Could you check a few things on this model? Use its own coordinates, in mm. Coordinates: 2 decimals unless noted, no trailing zeros. Order: outer loops, then holes, each group sorted by start corner. A loop starts at its lowest first (then second) coordinate and runs counter-clockwise, first axis right, second up. Notation, with made-up numbers: (-14, 52.25) -> (8, 52.25) arc R15 cw to (8, 81.25) -> close; hole circle Ø5 at (-23.5, 28). An arc over 180 degrees is marked (long way). Use a Markdown table: item, result. Add a question column.
1) If we section it at B-B (z = 2.65): Write out the boundary of the cut face in (x, y).
2) If we section it at A-A (x = 0): Write out the boundary of the cut face in (y, z), plus the area to 4 significant figures.
3) If we section it at D-D (z = 4.75): Write out the boundary of the cut face in (x, y), plus the area to 3 significant figures.
4) Will these pins go through, and if not, where does the flat tip stop? pin 1 Ø3 at (y, z) = (-12, 2) entering from -X; pin 2 Ø1 at (x, y) = (7, -14.5) entering from +Z.
5) If we section it at C-C (x = 14.5): Write out the boundary of the cut face in (y, z).
6) If I drill on L1, parallel to Y at x = 0, z = 0.6; L2, parallel to Y at x = -9.5, z = 0.35; L3, parallel to Z at x = -17.5, y = 2, over which ranges is the centre line in solid material (lowest first)? Write a range as [from, to].
```python
from build123d import *

# Parameters (mm, degrees)
CROQUIS2_R              = 20
SALIENTE_EXTRUIR2_DEPTH = 1
CROQUIS2_5_R            = 5
SALIENTE_EXTRUIR3_DEPTH = 5.5
CHAFL_N1_SIZE           = 5
CORTAR_EXTRUIR1_DEPTH   = 29.814059068


with BuildPart() as part:
    # Croquis2 → Saliente-Extruir2 (new body)
    with BuildSketch(Plane.XY):
        Circle(CROQUIS2_R)
        with BuildLine():
            Line((-2.039607805, 0.95), (2.039607805, 0.95))
            ThreePointArc((2.039607805, 0.95), (0, -2.25), (-2.039607805, 0.95))
        make_face(mode=Mode.SUBTRACT)
        with BuildLine():
            Line((-0.854679553, 13.973887178), (-1.098873712, 17.966426372))
            ThreePointArc((-1.098873712, 17.966426372), (0, 18), (1.098873712, 17.966426372))
            Line((1.098873712, 17.966426372), (0.854679553, 13.973887178))
            ThreePointArc((0.854679553, 13.973887178), (0, 14), (-0.854679553, 13.973887178))
        make_face(mode=Mode.SUBTRACT)
        with BuildLine():
            Line((-3.58862282, 17.638644683), (-2.791151082, 13.718945865))
            ThreePointArc((-2.791151082, 13.718945865), (-3.623466631, 13.522961568), (-4.44226519, 13.276531173))
            Line((-4.44226519, 13.276531173), (-5.711483815, 17.069825794))
            ThreePointArc((-5.711483815, 17.069825794), (-4.658742812, 17.386664873), (-3.58862282, 17.638644683))
        make_face(mode=Mode.SUBTRACT)
        with BuildLine():
            Line((-8.031560636, 16.108818509), (-6.246769384, 12.529081062))
            ThreePointArc((-6.246769384, 12.529081062), (-7, 12.124355653), (-7.727117794, 11.674401509))
            Line((-7.727117794, 11.674401509), (-9.934865736, 15.009944797))
            ThreePointArc((-9.934865736, 15.009944797), (-9, 15.588457268), (-8.031560636, 16.108818509))
        make_face(mode=Mode.SUBTRACT)
        with BuildLine():
            Line((-11.927160868, 13.481202974), (-9.276680675, 10.485380091))
            ThreePointArc((-9.276680675, 10.485380091), (-9.899494937, 9.899494937), (-10.485380091, 9.276680675))
            Line((-10.485380091, 9.276680675), (-13.481202974, 11.927160868))
            ThreePointArc((-13.481202974, 11.927160868), (-12.727922061, 12.727922061), (-11.927160868, 13.481202974))
        make_face(mode=Mode.SUBTRACT)
        with BuildLine():
            Line((-15.009944797, 9.934865736), (-11.674401509, 7.727117794))
            ThreePointArc((-11.674401509, 7.727117794), (-12.124355653, 7), (-12.529081062, 6.246769384))
            Line((-12.529081062, 6.246769384), (-16.108818509, 8.031560636))
            ThreePointArc((-16.108818509, 8.031560636), (-15.588457268, 9), (-15.009944797, 9.934865736))
        make_face(mode=Mode.SUBTRACT)
        with BuildLine():
            Line((-17.069825794, 5.711483815), (-13.276531173, 4.44226519))
            ThreePointArc((-13.276531173, 4.44226519), (-13.522961568, 3.623466631), (-13.718945865, 2.791151082))
            Line((-13.718945865, 2.791151082), (-17.638644683, 3.58862282))
            ThreePointArc((-17.638644683, 3.58862282), (-17.386664873, 4.658742812), (-17.069825794, 5.711483815))
        make_face(mode=Mode.SUBTRACT)
        with BuildLine():
            Line((-17.966426372, 1.098873712), (-13.973887178, 0.854679553))
            ThreePointArc((-13.973887178, 0.854679553), (-14, 0), (-13.973887178, -0.854679553))
            Line((-13.973887178, -0.854679553), (-17.966426372, -1.098873712))
            ThreePointArc((-17.966426372, -1.098873712), (-18, 0), (-17.966426372, 1.098873712))
        make_face(mode=Mode.SUBTRACT)
        with BuildLine():
            Line((-17.638644683, -3.58862282), (-13.718945865, -2.791151082))
            ThreePointArc((-13.718945865, -2.791151082), (-13.522961568, -3.623466631), (-13.276531173, -4.44226519))
            Line((-13.276531173, -4.44226519), (-17.069825794, -5.711483815))
            ThreePointArc((-17.069825794, -5.711483815), (-17.386664873, -4.658742812), (-17.638644683, -3.58862282))
        make_face(mode=Mode.SUBTRACT)
        with BuildLine():
            Line((-16.108818509, -8.031560636), (-12.529081062, -6.246769384))
            ThreePointArc((-12.529081062, -6.246769384), (-12.124355653, -7), (-11.674401509, -7.727117794))
            Line((-11.674401509, -7.727117794), (-15.009944797, -9.934865736))
            ThreePointArc((-15.009944797, -9.934865736), (-15.588457268, -9), (-16.108818509, -8.031560636))
        make_face(mode=Mode.SUBTRACT)
        with BuildLine():
            Line((-13.481202974, -11.927160868), (-10.485380091, -9.276680675))
            ThreePointArc((-10.485380091, -9.276680675), (-9.899494937, -9.899494937), (-9.276680675, -10.485380091))
            Line((-9.276680675, -10.485380091), (-11.927160868, -13.481202974))
            ThreePointArc((-11.927160868, -13.481202974), (-12.727922061, -12.727922061), (-13.481202974, -11.927160868))
        make_face(mode=Mode.SUBTRACT)
        with BuildLine():
            Line((-9.934865736, -15.009944797), (-7.727117794, -11.674401509))
            ThreePointArc((-7.727117794, -11.674401509), (-7, -12.124355653), (-6.246769384, -12.529081062))
            Line((-6.246769384, -12.529081062), (-8.031560636, -16.108818509))
            ThreePointArc((-8.031560636, -16.108818509), (-9, -15.588457268), (-9.934865736, -15.009944797))
        make_face(mode=Mode.SUBTRACT)
        with BuildLine():
            Line((-5.711483815, -17.069825794), (-4.44226519, -13.276531173))
            ThreePointArc((-4.44226519, -13.276531173), (-3.623466631, -13.522961568), (-2.791151082, -13.718945865))
            Line((-2.791151082, -13.718945865), (-3.58862282, -17.638644683))
            ThreePointArc((-3.58862282, -17.638644683), (-4.658742812, -17.386664873), (-5.711483815, -17.069825794))
        make_face(mode=Mode.SUBTRACT)
        with BuildLine():
            Line((-1.098873712, -17.966426372), (-0.854679553, -13.973887178))
            ThreePointArc((-0.854679553, -13.973887178), (0, -14), (0.854679553, -13.973887178))
            Line((0.854679553, -13.973887178), (1.098873712, -17.966426372))
            ThreePointArc((1.098873712, -17.966426372), (0, -18), (-1.098873712, -17.966426372))
        make_face(mode=Mode.SUBTRACT)
        with BuildLine():
            Line((3.58862282, -17.638644683), (2.791151082, -13.718945865))
            ThreePointArc((2.791151082, -13.718945865), (3.623466631, -13.522961568), (4.44226519, -13.276531173))
            Line((4.44226519, -13.276531173), (5.711483815, -17.069825794))
            ThreePointArc((5.711483815, -17.069825794), (4.658742812, -17.386664873), (3.58862282, -17.638644683))
        make_face(mode=Mode.SUBTRACT)
        with BuildLine():
            Line((8.031560636, -16.108818509), (6.246769384, -12.529081062))
            ThreePointArc((6.246769384, -12.529081062), (7, -12.124355653), (7.727117794, -11.674401509))
            Line((7.727117794, -11.674401509), (9.934865736, -15.009944797))
            ThreePointArc((9.934865736, -15.009944797), (9, -15.588457268), (8.031560636, -16.108818509))
        make_face(mode=Mode.SUBTRACT)
        with BuildLine():
            Line((11.927160868, -13.481202974), (9.276680675, -10.485380091))
            ThreePointArc((9.276680675, -10.485380091), (9.899494937, -9.899494937), (10.485380091, -9.276680675))
            Line((10.485380091, -9.276680675), (13.481202974, -11.927160868))
            ThreePointArc((13.481202974, -11.927160868), (12.727922061, -12.727922061), (11.927160868, -13.481202974))
        make_face(mode=Mode.SUBTRACT)
        with BuildLine():
            Line((15.009944797, -9.934865736), (11.674401509, -7.727117794))
            ThreePointArc((11.674401509, -7.727117794), (12.124355653, -7), (12.529081062, -6.246769384))
            Line((12.529081062, -6.246769384), (16.108818509, -8.031560636))
            ThreePointArc((16.108818509, -8.031560636), (15.588457268, -9), (15.009944797, -9.934865736))
        make_face(mode=Mode.SUBTRACT)
        with BuildLine():
            Line((17.069825794, -5.711483815), (13.276531173, -4.44226519))
            ThreePointArc((13.276531173, -4.44226519), (13.522961568, -3.623466631), (13.718945865, -2.791151082))
            Line((13.718945865, -2.791151082), (17.638644683, -3.58862282))
            ThreePointArc((17.638644683, -3.58862282), (17.386664873, -4.658742812), (17.069825794, -5.711483815))
        make_face(mode=Mode.SUBTRACT)
        with BuildLine():
            Line((17.966426372, -1.098873712), (13.973887178, -0.854679553))
            ThreePointArc((13.973887178, -0.854679553), (14, 0), (13.973887178, 0.854679553))
            Line((13.973887178, 0.854679553), (17.966426372, 1.098873712))
            ThreePointArc((17.966426372, 1.098873712), (18, 0), (17.966426372, -1.098873712))
        make_face(mode=Mode.SUBTRACT)
        with BuildLine():
            Line((17.638644683, 3.58862282), (13.718945865, 2.791151082))
            ThreePointArc((13.718945865, 2.791151082), (13.522961568, 3.623466631), (13.276531173, 4.44226519))
            Line((13.276531173, 4.44226519), (17.069825794, 5.711483815))
            ThreePointArc((17.069825794, 5.711483815), (17.386664873, 4.658742812), (17.638644683, 3.58862282))
        make_face(mode=Mode.SUBTRACT)
        with BuildLine():
            Line((16.108818509, 8.031560636), (12.529081062, 6.246769384))
            ThreePointArc((12.529081062, 6.246769384), (12.124355653, 7), (11.674401509, 7.727117794))
            Line((11.674401509, 7.727117794), (15.009944797, 9.934865736))
            ThreePointArc((15.009944797, 9.934865736), (15.588457268, 9), (16.108818509, 8.031560636))
        make_face(mode=Mode.SUBTRACT)
        with BuildLine():
            Line((13.481202974, 11.927160868), (10.485380091, 9.276680675))
            ThreePointArc((10.485380091, 9.276680675), (9.899494937, 9.899494937), (9.276680675, 10.485380091))
            Line((9.276680675, 10.485380091), (11.927160868, 13.481202974))
            ThreePointArc((11.927160868, 13.481202974), (12.727922061, 12.727922061), (13.481202974, 11.927160868))
        make_face(mode=Mode.SUBTRACT)
        with BuildLine():
            Line((9.934865736, 15.009944797), (7.727117794, 11.674401509))
            ThreePointArc((7.727117794, 11.674401509), (7, 12.124355653), (6.246769384, 12.529081062))
            Line((6.246769384, 12.529081062), (8.031560636, 16.108818509))
            ThreePointArc((8.031560636, 16.108818509), (9, 15.588457268), (9.934865736, 15.009944797))
        make_face(mode=Mode.SUBTRACT)
        with BuildLine():
            Line((5.711483815, 17.069825794), (4.44226519, 13.276531173))
            ThreePointArc((4.44226519, 13.276531173), (3.623466631, 13.522961568), (2.791151082, 13.718945865))
            Line((2.791151082, 13.718945865), (3.58862282, 17.638644683))
            ThreePointArc((3.58862282, 17.638644683), (4.658742812, 17.386664873), (5.711483815, 17.069825794))
        make_face(mode=Mode.SUBTRACT)
    extrude(amount=SALIENTE_EXTRUIR2_DEPTH)

    # Croquis2<5> → Saliente-Extruir3 (add)
    with BuildSketch(Plane.XY):
        Circle(CROQUIS2_5_R)
    extrude(amount=SALIENTE_EXTRUIR3_DEPTH)

    # Chaflán1
    # the kernel refuses this chamfer: 5 mm, written as the material it adds along each edge
    with BuildSketch(Plane(origin=(0, 0, 1), x_dir=(1, 0, 0), z_dir=(0, 1, 0))) as chafl_n1_piece_1_section:
        Polygon((5 + CHAFL_N1_SIZE, 0), (5, -CHAFL_N1_SIZE), (5, 0), align=None)
    chafl_n1_piece_1 = revolve(axis=Axis((0, 0, 1), (0, 0, -1)), mode=Mode.PRIVATE)
    chafl_n1_piece_1 = split(chafl_n1_piece_1, bisect_by=Plane(origin=(-7.762197096, 0, 5.5), z_dir=(0, 0, -1)), keep=Keep.TOP, mode=Mode.PRIVATE)
    add(chafl_n1_piece_1)

    # Croquis2<6> → Cortar-Extruir1 (cut, through all)
    with BuildSketch(Plane.XY):
        with BuildLine():
            Line((2.039607805, 0.95), (-2.039607805, 0.95))
            ThreePointArc((-2.039607805, 0.95), (-0.486509218, -2.196772355), (2.25, 0))
            ThreePointArc((2.25, 0), (2.196772355, 0.486509218), (2.039607805, 0.95))
        make_face()
    extrude(amount=CORTAR_EXTRUIR1_DEPTH, mode=Mode.SUBTRACT)


solid = part.part
```
Answer sheet:
| question | item | result |
|---|---|---|
| 1 | outline | circle Ø16.7 at (0, 0); hole (-2.04, 0.95) arc R2.25 ccw (long way) to (2.04, 0.95) -> close |
| 2 | outline | (-20, 0) -> (-18, 0) -> (-18, 1) -> (-20, 1) -> close; (-14, 0) -> (-2.25, 0) -> (-2.25, 5.5) -> (-5.5, 5.5) -> (-10, 1) -> (-14, 1) -> close; (0.95, 0) -> (14, 0) -> (14, 1) -> (10, 1) -> (5.5, 5.5) -> (0.95, 5.5) -> close; (18, 0) -> (20, 0) -> (20, 1) -> (18, 1) -> close |
| 2 | area | 84.15 mm2 |
| 3 | outline | circle Ø12.5 at (0, 0); hole (-2.04, 0.95) arc R2.25 ccw (long way) to (2.04, 0.95) -> close |
| 3 | area | 111 mm2 |
| 4 | pin 1 | x = -16.78 |
| 4 | pin 2 | z = 1 |
| 5 | outline | (-13.77, 0) -> (-9.6, 0) -> (-9.6, 1) -> (-13.77, 1) -> close; (-7.23, 0) -> (-4.85, 0) -> (-4.85, 1) -> (-7.23, 1) -> close; (-2.95, 0) -> (-0.89, 0) -> (-0.89, 1) -> (-2.95, 1) -> close; (0.89, 0) -> (2.95, 0) -> (2.95, 1) -> (0.89, 1) -> close; (4.85, 0) -> (7.23, 0) -> (7.23, 1) -> (4.85, 1) -> close; (9.6, 0) -> (13.77, 0) -> (13.77, 1) -> (9.6, 1) -> close |
| 6 | L1 | [-20, -18], [-14, -2.25], [0.95, 14], [18, 20] |
| 6 | L2 | [-17.6, -15.29], [-14.35, -10.74], [-10.28, 10.28], [10.74, 14.35], [15.29, 17.6] |
| 6 | L3 | [0, 1] |
